from build123d import *

# Parameters (mm, degrees)
CROQUIS1_R              = 8.35
SALIENTE_EXTRUIR1_DEPTH = 12.5
SALIENTE_EXTRUIR2_DEPTH = 10.5
CROQUIS3_R              = 8.35
CORTAR_EXTRUIR1_DEPTH   = 47


with BuildPart() as part:
    # Croquis1 → Saliente-Extruir1 (new, symmetric)
    with BuildSketch(Plane.XY):
        with BuildLine():
            Line((-11.35, 12), (11.35, 12))
            Line((11.35, 12), (11.35, 0))
            ThreePointArc((11.35, 0), (0, -11.35), (-11.35, 0))
            Line((-11.35, 0), (-11.35, 12))
        make_face()
        Circle(CROQUIS1_R, mode=Mode.SUBTRACT)
    extrude(amount=SALIENTE_EXTRUIR1_DEPTH, both=True)

    # Croquis2 → Saliente-Extruir2 (add, symmetric)
    with BuildSketch(Plane(origin=(0, 0, 0), x_dir=(0, 0, -1), z_dir=(1, 0, 0))):
        Polygon((-12.5, 12), (-12.5, 37), (1.642135624, 51.142135624), (15.784271247, 37), (2.716681877, 23.93241063), (4.090100333, 12), align=None)
    extrude(amount=SALIENTE_EXTRUIR2_DEPTH, both=True)

    # Croquis3 → Cortar-Extruir1 (cut)
    with BuildSketch(Plane(origin=(0, 26.392135624, -26.392135624), x_dir=(1, 0, 0), z_dir=(0, 0.7071067811865465, -0.7071067811865487))):
        with Locations(Location((0, -25.001785669, 0), (0, 0, 270))):
            Circle(CROQUIS3_R)
    extrude(amount=-CORTAR_EXTRUIR1_DEPTH, mode=Mode.SUBTRACT)


solid = part.part
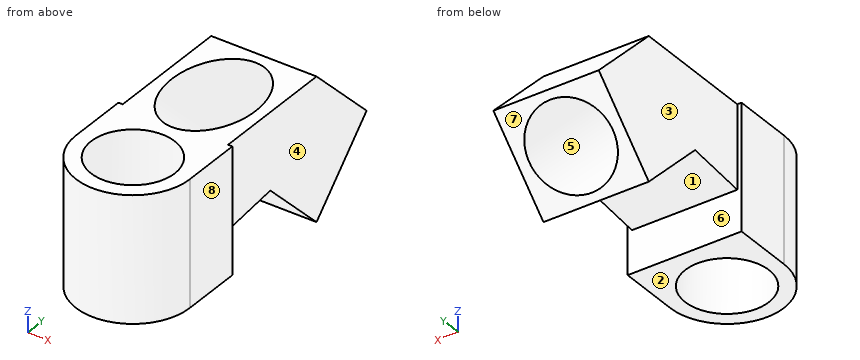
Could you check a few things on this model? Use its own coordinates, in mm. Face numbers are marked on the shaded views. A direction names the side the tool comes from. Give positions to 0.01 mm unless a question says otherwise; leave off trailing zeros. Write each loop counter-clockwise with the first axis right and the second up, starting at its lowest first coordinate (ties: lowest second). Pieces come first, ordered by that corner, then holes. Notation, with made-up numbers: (2, 6) - (33, 6) arc R15 cw to (33, 25) - close; hole circle Ø6 at (87, 16.5). An arc over 180 degrees is marked (long way). Use CSV: the item, a comma, the result in double quotes. Start each with the question number.
Item 1: I want a section at A-A, the plane x = 0. Please give me the cut outline in (y, z), then the cut area to 3 significant figures.
Item 2: If we mould it in two halves opening along Y, with no side actions, what happens to the marked faces 6, 7 and 8? For each: pulls with the +Y half, pulls with the -Y half, needs draft (parallel to the pull), parting line crosses it, or undercut.
Item 3: I want a section at B-B, the plane y = 2.5. Please give me the cut outline in (x, z).
Item 4: For the marked faces 1, 2, 3, 4 and 5, which set-ups out of +Z, -Z, +X, -X, +Y, -Y let a thin tool reach every point of the face, with its end or its side?
Item 5: If I drill on line 1 along Y through (x, z) = (4.5, 8); line 2 along Y through (x, z) = (3, -1.75); line 3 along X through (y, z) = (-7, -8), over which ranges is the centre line in solid material (lowest first)?
Item 6: I'm going to push flat-ended pins straight in: pin 1 (8 mm diameter, centred on x = 7.5, y = 37.5, fed in from -Z); pin 2 (2 mm diameter, centred on x = 3, z = -8, fed in from +Y); pin 3 (14 mm diameter, centred on y = 25, z = -4.5, fed in from -X); pin 4 (11.5 mm diameter, centred on x = -5, z = 4.5, fed in from +Y). Where does each tip first touch, or does it pass through?
Item 7: I want a section at C-C, the plane z = -6. Give the number of separate pieces and of enclosed holes in the cut face, then the cut area to 3 significant figures.
Item 8: I want a section at D-D, the plane x = 6.25. Please give me the cut outline in (y, z), then the cut area to 3 significant figures.
Findings:
1,outline,"(-11.35, -12.5) - (-8.35, -12.5) - (-8.35, 12.5) - (-11.35, 12.5) - close; (8.35, -12.5) - (12, -12.5) - (12, -4.09) - (23.93, -2.72) - (37, -15.78) - (38.17, -14.62) - (11.05, 12.5) - (8.35, 12.5) - close; (34.67, 12.5) - (49.98, -2.81) - (51.14, -1.64) - (37, 12.5) - close"
1,area,"339 mm2"
2,face 6,"undercut"
2,face 7,"pulls with the +Y half"
2,face 8,"needs draft"
3,outline,"(-11.35, -12.5) - (-7.97, -12.5) - (-7.97, 12.5) - (-11.35, 12.5) - close; (7.97, -12.5) - (11.35, -12.5) - (11.35, 12.5) - (7.97, 12.5) - close"
4,face 1,"-Z, +X, -X"
4,face 2,"-Z, +X, -X, -Y"
4,face 3,"+Z, -Z, -X, +Y"
4,face 4,"+Z, -Z, +X, +Y"
4,face 5,"none"
5,line 1,"y = -10.42 to -7.03, 7.03 to 17.41, 37.3 to 41.5"
5,line 2,"y = -10.95 to -7.79, 7.79 to 26.09, 48.13 to 51.03"
5,line 3,"x = -8.93 to -4.55, 4.55 to 8.93"
6,pin 1,"stops at z = -15.78"
6,pin 2,"stops at y = 33.5"
6,pin 3,"stops at x = -10.5"
6,pin 4,"stops at y = 50.75"
7,separate pieces,"2"
7,enclosed holes,"1"
7,area,"424 mm2"
8,outline,"(-9.47, -12.5) - (-5.54, -12.5) - (-5.54, 12.5) - (-9.47, 12.5) - close; (5.54, -12.5) - (12, -12.5) - (12, -4.09) - (23.93, -2.72) - (37, -15.78) - (40.16, -12.63) - (15.03, 12.5) - (5.54, 12.5) - close; (30.69, 12.5) - (47.99, -4.8) - (51.14, -1.64) - (37, 12.5) - close"
8,area,"602 mm2"
